Check sheet for the modelled part. Datum: model origin and axes. Units: mm. Give positions to 0.01 mm unless a question says otherwise; leave off trailing zeros. Loops run counter-clockwise (first coordinate to the right, second up) from the corner with the lowest first, then second, coordinate; pieces in that order, holes last. Notation, with made-up numbers: M -17,-17.5 L 9,-17.5 A31 cw 9,7.5 Z; hole C 48,75.5 d11. An arc over 180 degrees is marked long. Write each question's results on one line, items separated by ' | '. Start each with the question number.
1. Material ranges on line 1 along Z through (x, y) = (-135.5, 1); line 2 along Z through (x, y) = (-112, 1.7); line 3 along X through (y, z) = (1.75, -1), recorded low to high.
2. Go/stop test with flat-tipped pins: pin 1 (3.5 mm diameter, centred on x = 80.99, z = -110.28, fed in from +Y); pin 2 (1.5 mm diameter, centred on x = 110, z = -120, fed in from -Y); pin 3 (1.5 mm diameter, centred on x = -91.5, y = 1, fed in from +Z). Record where each tip stops, or that it passes through.
3. Sectioned sample at C-C on z = 76. Record the cut outline in (x, y).
4. Sectioned sample at A-A on y = 2.3. Give the number of separate pieces and of enclosed holes in the cut face, and give its area (3 significant figures).
5. Sectioned sample at B-B on x = -101. Record the cut outline in (y, z), and give its area (3 significant figures).
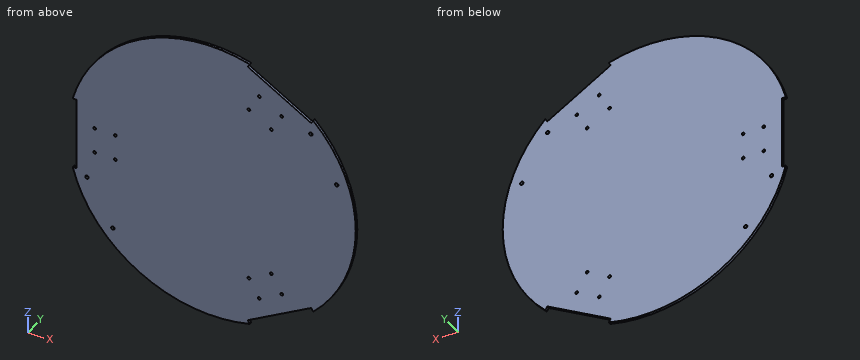
```python
from build123d import *

# Parameters (mm, degrees)
SKETCH_2_R               = 167
EXTRUDE_1_DEPTH          = 3
CUT_EXTRUDE_3_REACH      = 238.193
SKETCH_1_R               = 1.6
PATTERN_CIRCULAR_1_COUNT = 3
CUT_EXTRUDE_4_REACH      = 238.193
SKETCH_3_W               = 90.124680173
SKETCH_3_H               = 85
PATTERN_CIRCULAR_2_COUNT = 3
SKETCH_4_R               = 2
CUT_EXTRUDE_5_DEPTH      = 10
MIRROR_2_COPY_1_SKETCH_R = 2
MIRROR_2_COPY_1_DEPTH    = 10


with BuildPart() as part:
    # Sketch 2 → Extrude 1 (new body)
    with BuildSketch(Plane(origin=(0, 0, 0), x_dir=(1, 0, 0), z_dir=(0, 1, 0))):
        with Locations(Location((0, 0, 0), (0, 0, 270))):
            Circle(SKETCH_2_R)
    extrude(amount=EXTRUDE_1_DEPTH)

    # Sketch 1 → Cut-Extrude 3 (cut, up to next)
    with BuildSketch(Plane(origin=(0, 0, 0), x_dir=(1, 0, 0), z_dir=(0, 1, 0)), mode=Mode.PRIVATE) as cut_extrude_3_sk1:
        with Locations(Location((-112, 15, 0), (0, 0, 90))):
            Circle(SKETCH_1_R)
    cut_extrude_3_tool1 = extrude(cut_extrude_3_sk1.sketch, amount=CUT_EXTRUDE_3_REACH, mode=Mode.PRIVATE) & part.part
    # Sketch 1 → Cut-Extrude 3 (cut, up to next)
    with BuildSketch(Plane(origin=(0, 0, 0), x_dir=(1, 0, 0), z_dir=(0, 1, 0)), mode=Mode.PRIVATE) as cut_extrude_3_sk2:
        with Locations(Location((-112, -15, 0), (0, 0, 90))):
            Circle(SKETCH_1_R)
    cut_extrude_3_tool2 = extrude(cut_extrude_3_sk2.sketch, amount=CUT_EXTRUDE_3_REACH, mode=Mode.PRIVATE) & part.part
    # Sketch 1 → Cut-Extrude 3 (cut, up to next)
    with BuildSketch(Plane(origin=(0, 0, 0), x_dir=(1, 0, 0), z_dir=(0, 1, 0)), mode=Mode.PRIVATE) as cut_extrude_3_sk3:
        with Locations(Location((-136, 15, 0), (0, 0, 90))):
            Circle(SKETCH_1_R)
    cut_extrude_3_tool3 = extrude(cut_extrude_3_sk3.sketch, amount=CUT_EXTRUDE_3_REACH, mode=Mode.PRIVATE) & part.part
    # Sketch 1 → Cut-Extrude 3 (cut, up to next)
    with BuildSketch(Plane(origin=(0, 0, 0), x_dir=(1, 0, 0), z_dir=(0, 1, 0)), mode=Mode.PRIVATE) as cut_extrude_3_sk4:
        with Locations(Location((-136, -15, 0), (0, 0, 90))):
            Circle(SKETCH_1_R)
    cut_extrude_3_tool4 = extrude(cut_extrude_3_sk4.sketch, amount=CUT_EXTRUDE_3_REACH, mode=Mode.PRIVATE) & part.part
    cut_extrude_3_1 = cut_extrude_3_tool1.solids().sort_by_distance((-112, 0, -15))[0]
    add(cut_extrude_3_1, mode=Mode.SUBTRACT)
    cut_extrude_3_2 = cut_extrude_3_tool2.solids().sort_by_distance((-112, 0, 15))[0]
    add(cut_extrude_3_2, mode=Mode.SUBTRACT)
    cut_extrude_3_3 = cut_extrude_3_tool3.solids().sort_by_distance((-136, 0, -15))[0]
    add(cut_extrude_3_3, mode=Mode.SUBTRACT)
    cut_extrude_3_4 = cut_extrude_3_tool4.solids().sort_by_distance((-136, 0, 15))[0]
    add(cut_extrude_3_4, mode=Mode.SUBTRACT)
    cut_extrude_3 = cut_extrude_3_1 + cut_extrude_3_2 + cut_extrude_3_3 + cut_extrude_3_4  # Cut-Extrude 3 as one shape, for the pattern or mirror that repeats it

    # Pattern Circular 1: Cut-Extrude 3 ×3 about axis
    pattern_circular_1_axis = Axis((0, 0, 0), (0, 1, 0))
    for i in range(1, PATTERN_CIRCULAR_1_COUNT):
        add(cut_extrude_3.rotate(pattern_circular_1_axis, i * 360 / PATTERN_CIRCULAR_1_COUNT), mode=Mode.SUBTRACT)

    # Sketch 3 → Cut-Extrude 4 (cut, up to next)
    with BuildSketch(Plane(origin=(0, 3, 0), x_dir=(1, 0, 0), z_dir=(0, 1, 0)), mode=Mode.PRIVATE) as cut_extrude_4_sk1:
        with Locations((-202.062340087, 0)):
            Rectangle(SKETCH_3_W, SKETCH_3_H)
    cut_extrude_4_tool1 = extrude(cut_extrude_4_sk1.sketch, amount=-CUT_EXTRUDE_4_REACH, mode=Mode.PRIVATE) & part.part
    cut_extrude_4 = cut_extrude_4_tool1.solids().sort_by_distance((-202.06234, 3, 0))[0]
    add(cut_extrude_4, mode=Mode.SUBTRACT)

    # Pattern Circular 2: Cut-Extrude 4 ×3 about axis
    pattern_circular_2_axis = Axis((0, 0, 0), (0, 1, 0))
    for i in range(1, PATTERN_CIRCULAR_2_COUNT):
        add(cut_extrude_4.rotate(pattern_circular_2_axis, i * 360 / PATTERN_CIRCULAR_2_COUNT), mode=Mode.SUBTRACT)

    # Sketch 4 → Cut-Extrude 5 (cut)
    with BuildSketch(Plane.XZ):
        with Locations(Location((-144.903810568, -49.019237886, 0), (0, 0, 270))):
            Circle(SKETCH_4_R)
    cut_extrude_5 = extrude(amount=-CUT_EXTRUDE_5_DEPTH, mode=Mode.SUBTRACT)

    # Mirror 1: Cut-Extrude 5 across plane
    add(cut_extrude_5.mirror(Plane(origin=(0, 0, 0), x_dir=(0.8660254037844363, 0, 0.500000000000004), z_dir=(0.5000000000000042, 0, -0.8660254037844363))), mode=Mode.SUBTRACT)

    # Mirror 2: Cut-Extrude 5 across plane
    add(cut_extrude_5.mirror(Plane(origin=(0, 0, 0), x_dir=(-0.500000000000004, 0, 0.8660254037844363), z_dir=(-0.8660254037844365, 0, -0.500000000000004))), mode=Mode.SUBTRACT)

    # Mirror 2 copy 1 sketch → Mirror 2 copy 1 (cut)
    with BuildSketch(Plane(origin=(0, 0, 0), x_dir=(-1, 0, 0), z_dir=(0, -1, 0))):
        with Locations(Location((-144.903810568, -49.019237886, 0), (0, 0, 270))):
            Circle(MIRROR_2_COPY_1_SKETCH_R)
    extrude(amount=-MIRROR_2_COPY_1_DEPTH, mode=Mode.SUBTRACT)


solid = part.part
```
Output values:
1) line 1: -97.62 to -16.52, -13.48 to 13.48, 16.52 to 97.62 | line 2: -123.87 to -16.6, -13.4 to 13.4, 16.6 to 123.87 | line 3: -157 to 167
2) pin 1: y = 3 | pin 2: through | pin 3: z = 140.19
3) outline: M -148.7,0 L 148.7,0 L 148.7,3 L -148.7,3 Z
4) separate pieces: 1 | enclosed holes: 16 | area: 85,400 mm2
5) outline: M 0,-133 L 3,-133 L 3,133 L 0,133 Z | area: 798 mm2
